Here's how the part is built. I have some questions about the finished solid (model axes, mm). Face numbers are marked on the shaded views. A direction names the side the tool comes from. Give positions to 0.01 mm unless a question says otherwise; leave off trailing zeros. Write each loop counter-clockwise with the first axis right and the second up, starting at its lowest first coordinate (ties: lowest second). Pieces come first, ordered by that corner, then holes. Notation, with made-up numbers: (43, -0.75) -> (61, -0.75) arc R14 ccw to (61, 17.25) -> close; hole circle Ø10 at (-25.75, 12). An arc over 180 degrees is marked (long way). Use CSV: the item, a comma, the result in double quotes. Start each with the question number.
(1) Suppose I cut it at A-A on z = 1.1. Give the number of separate pieces and of enclosed holes in the cut face, plus the area to 3 significant figures.
(2) For pin 1 Ø0.5 at (x, y) = (6, 1) entering from +Z, with a flat end and sliding along its axis, tell me the tip position at first contact or that it passes through.
(3) Suppose I cut it at C-C on x = 1.2. List the corners of the cut face in (y, z) for me, plus the area to 3 significant figures.
(4) If we mould it in two halves opening along X, with no side actions, what happens to the marked faces 1, 2 and 3? For each: pulls with the +X half, pulls with the -X half, needs draft (parallel to the pull), parting line crosses it, or undercut.
(5) Suppose I cut it at D-D on x = 7.1. List the corners of the cut face in (y, z) for me.
(6) Suppose I cut it at B-B on y = -0.1. List the corners of the cut face in (x, z) for me, plus the area to 3 significant figures.
(7) I need wall thicknesses on L1, parallel to X at y = 3.5, z = 0.55; L2, parallel to Y at x = 7.75, z = 0.85; L3, parallel to Y at x = 7.6, z = 0.65. Which ranges of each line are inside material? Lowest first, please. Write a range as [from, to].
(8) Which directions (+Z, -Z, +X, -X, +Y, -Y) give clear straight access to the entire face, cutting with the end or side of a thin tool? Please do the marked faces 4, 5, 6 and 7.
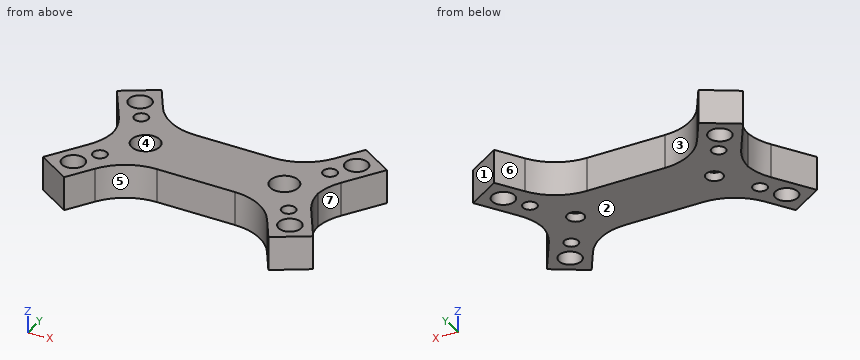
from build123d import *

# Parameters (mm, degrees)
BOSS_EXTRUDE1_DEPTH        = 1.2
HOLE1_D                    = 0.6
HOLE1_CBORE_D              = 1
HOLE1_CBORE_DEPTH          = 0.9
FILLET1_R                  = 2
F_0_8_0_8_DIAMETER_HOLE1_D = 0.8
F_0_5_0_5_DIAMETER_HOLE1_D = 0.5


with BuildPart() as part:
    # Sketch1 → Boss-Extrude1 (new body)
    with BuildSketch(Plane.XY.offset(1.2)):
        Polygon((0.021444953, -1.865705812), (1.187267335, 0), (6.212732665, 0), (7.378555047, -1.865705812), (8.565822381, -1.123818842), (7.4, 0.74188697), (7.4, 1.65811303), (8.565822381, 3.523818842), (7.378555047, 4.265705812), (6.212732665, 2.4), (1.187267335, 2.4), (0.021444953, 4.265705812), (-1.165822381, 3.523818842), (0, 1.65811303), (0, 0.74188697), (-1.165822381, -1.123818842), align=None)
    extrude(amount=-BOSS_EXTRUDE1_DEPTH)

    # Hole1 (through all)
    with Locations(Plane.XY.offset(1.2)):
        with Locations((1.2, 1.2), (6.2, 1.2)):
            CounterBoreHole(HOLE1_D / 2, HOLE1_CBORE_D / 2, HOLE1_CBORE_DEPTH)

    # Fillet1
    # the kernel refuses this fillet: 2 mm, written as the material it adds along each edge
    with BuildSketch(Plane(origin=(6.212732665, 2.4, 1.2), x_dir=(-1, 0, 0), z_dir=(0, 0, -1)), Plane(origin=(1.187267335, 2.4, 1.2), x_dir=(-0.5299192642332093, 0.8480480961564231, 0), z_dir=(0, 0, -1))) as fillet1_piece_1:
        with BuildLine():
            CenterArc((FILLET1_R * 0.554309051453, FILLET1_R), FILLET1_R, 212, 58)
            Line((-FILLET1_R * 0.293739044704, FILLET1_R * 0.470080735767), (0, 0))
            Line((0, 0), (FILLET1_R * 0.554309051453, 0))
        make_face()
    extrude(amount=1.2)
    with BuildSketch(Plane(origin=(7.4, 1.65811303, 1.2), x_dir=(0, -1, 0), z_dir=(0, 0, -1)), Plane(origin=(7.4, 0.74188697, 1.2), x_dir=(0.5299192642332092, -0.8480480961564232, 0), z_dir=(0, 0, -1))) as fillet1_piece_2:
        with BuildLine():
            CenterArc((FILLET1_R * 0.286745385759, -FILLET1_R), FILLET1_R, 90, 32)
            Line((-FILLET1_R * 0.243173878474, -FILLET1_R * 0.151951903844), (0, 0))
            Line((0, 0), (FILLET1_R * 0.286745385759, 0))
        make_face()
    extrude(amount=1.2)
    with BuildSketch(Plane(origin=(6.212732665, 0, 1.2), x_dir=(-1, 0, 0), z_dir=(0, 0, -1)), Plane(origin=(1.187267335, 0, 1.2), x_dir=(-0.5299192642332091, -0.8480480961564235, 0), z_dir=(0, 0, -1))) as fillet1_piece_3:
        with BuildLine():
            CenterArc((FILLET1_R * 0.554309051453, -FILLET1_R), FILLET1_R, 90, 58)
            Line((-FILLET1_R * 0.293739044704, -FILLET1_R * 0.470080735767), (0, 0))
            Line((0, 0), (FILLET1_R * 0.554309051453, 0))
        make_face()
    extrude(amount=1.2)
    with BuildSketch(Plane(origin=(0, 0.74188697, 1.2), x_dir=(-0.5299192642332088, -0.8480480961564235, 0), z_dir=(0, 0, -1)), Plane(origin=(0, 1.65811303, 1.2), x_dir=(0, -1, 0), z_dir=(0, 0, -1))) as fillet1_piece_4:
        with BuildLine():
            CenterArc((FILLET1_R * 0.286745385759, FILLET1_R), FILLET1_R, 238, 32)
            Line((-FILLET1_R * 0.243173878474, FILLET1_R * 0.151951903844), (0, 0))
            Line((0, 0), (FILLET1_R * 0.286745385759, 0))
        make_face()
    extrude(amount=1.2)

    # Ø0.8 (0.8) Diameter Hole1 (through all)
    with Locations(Plane.XY.offset(1.2)):
        with Locations((-0.2, 3.3), (7.6, 3.3), (-0.2, -0.9), (7.6, -0.9)):
            Hole(F_0_8_0_8_DIAMETER_HOLE1_D / 2)

    # Ø0.5 (0.5) Diameter Hole1 (through all)
    with Locations(Plane.XY.offset(1.2)):
        with Locations((7.1, -0.1), (0.3, -0.1), (0.3, 2.5), (7.1, 2.5)):
            Hole(F_0_5_0_5_DIAMETER_HOLE1_D / 2)


solid = part.part
Geometry says:
1,separate pieces,"1"
1,enclosed holes,"10"
1,area,"24.8 mm²"
2,pin 1,"z = 1.2"
3,outline,"(-0.33, 0) -> (0.9, 0) -> (0.9, 0.3) -> (0.7, 0.3) -> (0.7, 1.2) -> (-0.33, 1.2) -> close; (1.5, 0) -> (2.73, 0) -> (2.73, 1.2) -> (1.7, 1.2) -> (1.7, 0.3) -> (1.5, 0.3) -> close"
3,area,"2.58 mm²"
4,face 1,"pulls with the +X half"
4,face 2,"needs draft"
4,face 3,"undercut"
5,outline,"(-1.42, 0) -> (-0.35, 0) -> (-0.35, 1.2) -> (-1.42, 1.2) -> close; (0.15, 0) -> (2.25, 0) -> (2.25, 1.2) -> (0.15, 1.2) -> close; (2.75, 0) -> (3.82, 0) -> (3.82, 1.2) -> (2.75, 1.2) -> close"
6,outline,"(-0.53, 0) -> (0.05, 0) -> (0.05, 1.2) -> (-0.53, 1.2) -> close; (0.55, 0) -> (1.67, 0) -> (1.67, 1.2) -> (0.55, 1.2) -> close; (5.73, 0) -> (6.85, 0) -> (6.85, 1.2) -> (5.73, 1.2) -> close; (7.35, 0) -> (7.93, 0) -> (7.93, 1.2) -> (7.35, 1.2) -> close"
6,area,"4.07 mm²"
7,L1,"[-1.15, -0.55], [0.15, 0.5], [6.9, 7.25], [7.95, 8.55]"
7,L2,"[-1.63, -1.27], [-0.53, 0.18], [2.22, 2.93], [3.67, 4.03]"
7,L3,"[-1.73, -1.3], [-0.5, 0.44], [1.96, 2.9], [3.7, 4.13]"
8,face 4,"+Z"
8,face 5,"+Z, -Z, -Y"
8,face 6,"+Z, -Z, +Y"
8,face 7,"+Z, -Z, +X"
